Autodesk Inventor part; units mm, degrees
ref_plane "YZ Plane" through (0, 0, 0) normal (1, 0, 0) x (0, 1, 0)
ref_plane "XZ Plane" through (0, 0, 0) normal (0, 1, 0) x (-1, 0, 0)
ref_plane "XY Plane" through (0, 0, 0) normal (0, 0, 1) x (1, 0, 0)
sketch "Skizze1" plane through (0, 0, 0) normal (0, 0, 1) x (1, 0, 0)
  line L0 (-50.8, 50.8) -> (50.8, 50.8)
  line L1 (50.8, 50.8) -> (50.8, -50.8)
  line L2 (50.8, -50.8) -> (-50.8, -50.8)
  line L3 (-50.8, -50.8) -> (-50.8, 50.8)
  line L4 (50.8, -50.8) -> (-50.8, 50.8) construction
  point P0 (0, 0)
  point P1 (0, 0)
  dimension "d0" = 101.6
  dimension "d1" = 101.6
extrude "Extrusion1" add sketch "Skizze1" against normal blind 2.0066
fillet "Rundung1" radius 2.0066 4 edges at (50.8, -50.8, -1.0033) (50.8, 50.8, -1.0033) (-50.8, 50.8, -1.0033) (-50.8, -50.8, -1.0033)
fillet "Rundung2" radius 2.0066 8 edges at (-50.2123, -50.2123, -2.0066) (-50.8, 0, -2.0066) (-50.2123, 50.2123, -2.0066) (0, 50.8, -2.0066) (50.2123, 50.2123, -2.0066) (50.8, 0, -2.0066) (50.2123, -50.2123, -2.0066) (0, -50.8, -2.0066)
sketch "Skizze2" plane through (0, 0, 0) normal (0, 0, 1) x (1, 0, 0)
  line L0 (-47.5996, 47.5996) -> (47.5996, 47.5996)
  line L1 (47.5996, 47.5996) -> (47.5996, -47.5996)
  line L2 (47.5996, -47.5996) -> (-47.5996, -47.5996)
  line L3 (-47.5996, -47.5996) -> (-47.5996, 47.5996)
  line L4 (47.5996, -47.5996) -> (-47.5996, 47.5996) construction
  line L5 (-45.593, 45.593) -> (45.593, 45.593)
  line L6 (45.593, 45.593) -> (45.593, -45.593)
  line L7 (45.593, -45.593) -> (-45.593, -45.593)
  line L8 (-45.593, -45.593) -> (-45.593, 45.593)
  line L9 (-45.593, -45.593) -> (45.593, 45.593) construction
  point P0 (0, 0)
  point P1 (0, 0)
  dimension "d6" = 95.1992
  dimension "d7" = 2.0066
extrude "Extrusion2" add sketch "Skizze2" along normal blind 9.9822
sketch "Skizze3" plane through (47.5996, -47.5996, 0) normal (1, 0, 0) x (0, 0, -1)
  line L0 (0, 95.1992) -> (0, 0)
  line L1 (0, 95.1992) -> (-9.9822, 95.1992)
  line L2 (-9.9822, 0) -> (-9.9822, 95.1992)
  line L3 (0, 0) -> (-9.9822, 0)
  line L4 (0, 47.5996) -> (-4.7752, 47.5996) construction
  line L5 (0, 95.1992) -> (0, 0) construction
  dimension "d10" = 4.7752
hole "Bohrung1" at (47.5996, 0, 4.7752) direction (-1, 0, 0) diameter 1.941 depth 7.675 tip angle 118
pattern_circular "Runde Anordnung1" count 3 over 180 about axis through (0, 0, -10) along (0, 0, 1) of "Bohrung1"
sketch "Skizze4" plane through (-47.5996, -47.5996, 0) normal (0, -1, 0) x (1, 0, 0)
  line L0 (95.1992, 0) -> (0, 0)
  line L1 (95.1992, 0) -> (95.1992, 9.9822)
  line L2 (0, 9.9822) -> (95.1992, 9.9822)
  line L3 (0, 0) -> (0, 9.9822)
  line L4 (47.5996, 0) -> (47.5996, 4.7752) construction
  line L5 (28.5496, 4.7752) -> (66.6496, 4.7752) construction
  dimension "d21" = 4.7752
  dimension "d22" = 38.1
hole "Bohrung2" at (-19.05, -47.5996, 4.7752) at (19.05, -47.5996, 4.7752) direction (0, 1, 0) diameter 1.941 depth 7.675 tip angle 118
properties part number "Nanolab CubeDeckel 1"
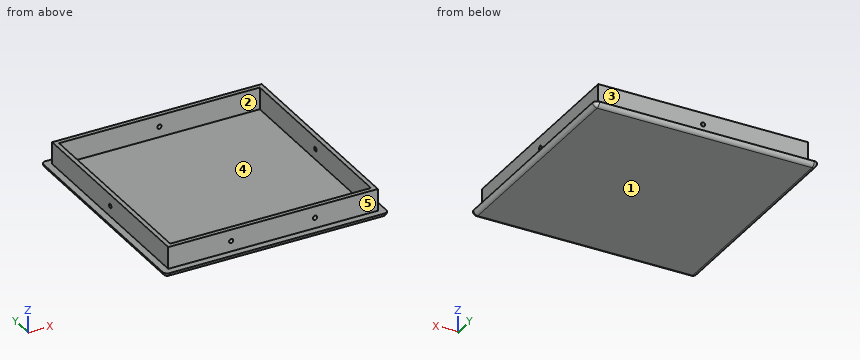
Check sheet for the modelled part. Datum: model origin and axes. Units: mm. Face numbers are marked on the shaded views. A direction names the side the tool comes from. Give positions to 0.01 mm unless a question says otherwise; leave off trailing zeros. Order: outer loops, then holes, each group sorted by start corner. A loop starts at its lowest first (then second) coordinate and runs counter-clockwise, first axis right, second up. Notation, with made-up numbers: (-8.5, 48) -> (17.5, 48) arc R18 cw to (17.5, 81) -> close; hole circle Ø10 at (12.25, 89). An arc over 180 degrees is marked (long way). Return JSON: item names as keys, results as strings.
1. Material ranges on probe 1 along X at (y, z) = (34, 3.75); probe 2 along Z at (x, y) = (-19, -46), recorded low to high. Write a range as [from, to].
From the geometry:
{"probe 1": "[-47.6, -45.59], [45.59, 47.6]", "probe 2": "[-2.01, 3.81], [5.74, 9.98]"}
2. Mould release check, pull along Y, two halves, no side actions. Record for the marked faces 3, 4 and 5: +Y half, -Y half, draft (parallel to the pull), parting line (faces both ways), or undercut.
From the geometry:
{"face 3": "+Y half", "face 4": "undercut", "face 5": "-Y half"}
3. Cross-section at B-B, the plane z = 8.75. Record the cut outline in (x, y), plus the area to 3 significant figures.
From the geometry:
{"outline": "(-47.6, -47.6) -> (47.6, -47.6) -> (47.6, 47.6) -> (-47.6, 47.6) -> close; hole (-45.59, -45.59) -> (45.59, -45.59) -> (45.59, 45.59) -> (-45.59, 45.59) -> close", "area": "748 mm^2"}
4. Set-up check for the marked faces 1 and 2: record each of +Z, -Z, +X, -X, +Y, -Y from which the full face is reachable in a straight line by a thin tool's end or side.
From the geometry:
{"face 1": "-Z, +X, -X, +Y, -Y", "face 2": "+Z"}
5. Go/stop test with flat-tipped pins: P1, Ø2.5, axis at x = -19.05, z = 4.78, coming from the +Y side; P2, Ø2, axis at y = 0, z = 4.78, coming from the +X side; P3, Ø8, axis at x = 18.5, y = 16, coming from the +Z side. Record where each tip stops, or that it passes through.
From the geometry:
{"P1": "y = 47.6", "P2": "x = 47.6", "P3": "z = 0"}
